from build123d import *

# Parameters (mm, degrees)
BOSS_EXTRUDE1_DEPTH = 17.018
BOSS_EXTRUDE2_DEPTH = 2.54
BOSS_EXTRUDE3_DEPTH = 6.35
SKETCH4_4_R         = 2.75
BOSS_EXTRUDE4_DEPTH = 10.414


with BuildPart() as part:
    # Sketch2 → Boss-Extrude1 (new body)
    with BuildSketch(Plane(origin=(0, 0, 0), x_dir=(1, 0, 0), z_dir=(0, 1, 0))):
        with BuildLine():
            Line((1.5, 0), (21.5, 0))
            ThreePointArc((21.5, 0), (22.560660172, -0.439339828), (23, -1.5))
            Line((23, -1.5), (23, -11.5))
            ThreePointArc((23, -11.5), (22.560660172, -12.560660172), (21.5, -13))
            Line((21.5, -13), (1.5, -13))
            ThreePointArc((1.5, -13), (0.439339828, -12.560660172), (0, -11.5))
            Line((0, -11.5), (0, -1.5))
            ThreePointArc((0, -1.5), (0.439339828, -0.439339828), (1.5, 0))
        make_face()
    extrude(amount=BOSS_EXTRUDE1_DEPTH)

    # Sketch3 → Boss-Extrude2 (add)
    with BuildSketch(Plane(origin=(0, 17.018, 0), x_dir=(1, 0, 0), z_dir=(0, 1, 0))):
        with BuildLine():
            Line((21.5, 0), (1.5, 0))
            ThreePointArc((1.5, 0), (0.439339828, -0.439339828), (0, -1.5))
            Line((0, -1.5), (0, -11.5))
            ThreePointArc((0, -11.5), (0.439339828, -12.560660172), (1.5, -13))
            Line((1.5, -13), (21.5, -13))
            ThreePointArc((21.5, -13), (22.560660172, -12.560660172), (23, -11.5))
            Line((23, -11.5), (23, -1.5))
            ThreePointArc((23, -1.5), (22.560660172, -0.439339828), (21.5, 0))
        make_face()
        with BuildLine():
            Line((0, -11.5), (0, -6.5))
            ThreePointArc((0, -6.5), (-0.557961582, -7.847038418), (-1.905, -8.405))
            Line((-1.905, -8.405), (-3.359, -8.405))
            Line((-3.359, -8.405), (-3.359, -11.5))
            ThreePointArc((-3.359, -11.5), (-2.919660172, -12.560660172), (-1.859, -13))
            Line((-1.859, -13), (1.5, -13))
            ThreePointArc((1.5, -13), (0.439339828, -12.560660172), (0, -11.5))
        make_face()
        with BuildLine():
            Line((1.5, 0), (-1.859, 0))
            ThreePointArc((-1.859, 0), (-2.919660172, -0.439339828), (-3.359, -1.5))
            Line((-3.359, -1.5), (-3.359, -4.595))
            Line((-3.359, -4.595), (-1.905, -4.595))
            ThreePointArc((-1.905, -4.595), (-0.557961582, -5.152961582), (0, -6.5))
            Line((0, -6.5), (0, -1.5))
            ThreePointArc((0, -1.5), (0.439339828, -0.439339828), (1.5, 0))
        make_face()
        with BuildLine():
            ThreePointArc((24.905, -8.405), (23.557961582, -7.847038418), (23, -6.5))
            Line((23, -6.5), (23, -11.5))
            ThreePointArc((23, -11.5), (22.560660172, -12.560660172), (21.5, -13))
            Line((21.5, -13), (24.859, -13))
            ThreePointArc((24.859, -13), (25.919660172, -12.560660172), (26.359, -11.5))
            Line((26.359, -11.5), (26.359, -8.405))
            Line((26.359, -8.405), (24.905, -8.405))
        make_face()
        with BuildLine():
            Line((24.859, 0), (21.5, 0))
            ThreePointArc((21.5, 0), (22.560660172, -0.439339828), (23, -1.5))
            Line((23, -1.5), (23, -6.5))
            ThreePointArc((23, -6.5), (23.557961582, -5.152961582), (24.905, -4.595))
            Line((24.905, -4.595), (26.359, -4.595))
            Line((26.359, -4.595), (26.359, -1.5))
            ThreePointArc((26.359, -1.5), (25.919660172, -0.439339828), (24.859, 0))
        make_face()
    extrude(amount=BOSS_EXTRUDE2_DEPTH)

    # Sketch4 → Boss-Extrude3 (add)
    with BuildSketch(Plane(origin=(0, 19.558, 0), x_dir=(1, 0, 0), z_dir=(0, 1, 0))):
        with BuildLine():
            Line((1.5, 0), (21.5, 0))
            ThreePointArc((21.5, 0), (22.560660172, -0.439339828), (23, -1.5))
            Line((23, -1.5), (23, -11.5))
            ThreePointArc((23, -11.5), (22.560660172, -12.560660172), (21.5, -13))
            Line((21.5, -13), (1.5, -13))
            ThreePointArc((1.5, -13), (0.439339828, -12.560660172), (0, -11.5))
            Line((0, -11.5), (0, -1.5))
            ThreePointArc((0, -1.5), (0.439339828, -0.439339828), (1.5, 0))
        make_face()
    extrude(amount=BOSS_EXTRUDE3_DEPTH)

    # Sketch4_4 → Boss-Extrude4 (add)
    with BuildSketch(Plane(origin=(0, 19.558, 0), x_dir=(1, 0, 0), z_dir=(0, 1, 0))):
        with Locations(Location((17.158, -6.5, 0), (0, 0, 270))):
            Circle(SKETCH4_4_R)
    extrude(amount=BOSS_EXTRUDE4_DEPTH)


solid = part.part
Input: part model. Units: mm. Frame: model coordinates. A direction names the side the tool comes from. Give positions to 0.01 mm unless a question says otherwise; leave off trailing zeros. Order: outer loops, then holes, each group sorted by start corner. A loop starts at its lowest first (then second) coordinate and runs counter-clockwise, first axis right, second up. Notation, with made-up numbers: M -1,-2 L 51,-2 A21 ccw 51,17 Z; hole C 71.25,31.25 d1. An arc over 180 degrees is marked long. Answer as a JSON object with one key per item and string values.
1. Cut plane B-B, the plane y = 16.5. Output: boundary loops of the cut face in (x, z).
Result sheet:
{"outline": "M 0,1.5 A1.5 ccw 1.5,0 L 21.5,0 A1.5 ccw 23,1.5 L 23,11.5 A1.5 ccw 21.5,13 L 1.5,13 A1.5 ccw 0,11.5 Z"}
2. Reachability of faces 4 (the flat face through (0, 23, 7)), 5 (the cylindrical face through (0.45, 8.39, 12.57)), 6 (the cylindrical face through (22.55, 22.69, 0.43)) from +Z, -Z, +X, -X, +Y, -Y: full face, straight path, thin tool, end or side. Return the list, or none.
Result sheet:
{"face 4": "+Z, -Z, -X, +Y", "face 5": "+Z, -X, -Y", "face 6": "-Z, +X, +Y"}
3. Cut plane D-D, the plane z = 7.25. Output: boundary loops of the cut face in (x, y).
Result sheet:
{"outline": "M -0.15,17.02 L 0,17.02 L 0,0 L 23,0 L 23,17.02 L 23.15,17.02 L 23.15,19.56 L 23,19.56 L 23,25.91 L 19.8,25.91 L 19.8,29.97 L 14.51,29.97 L 14.51,25.91 L 0,25.91 L 0,19.56 L -0.15,19.56 Z"}
4. First-contact query: P1, Ø1.5, axis at x = -1, z = 2, coming from the +Y side; P2, Ø3, axis at y = 24, z = 7.5, coming from the -X side; P3, Ø2, axis at y = 4, z = 8.5, coming from the +X side. Flat tips, straight axial feed; report the tip coordinate or a pass-through.
Result sheet:
{"P1": "y = 19.56", "P2": "x = 0", "P3": "x = 23"}
5. Pull-direction query (Z, two-part tool) for faces 1 (the flat face through (26.359, 18, 10)), 2 (the flat face through (26, 18, 4.595)), 3 (the cylindrical face through (22.55, 8.39, 0.43)); classes: +Z half, -Z half, draft (parallel to the pull), parting line (faces both ways), or undercut.
Result sheet:
{"face 1": "draft", "face 2": "undercut", "face 3": "-Z half"}
6. Cut plane C-C, the plane x = 12. Output: boundary loops of the cut face in (y, z), and give its area (3 significant figures).
Result sheet:
{"outline": "M 0,0 L 25.91,0 L 25.91,13 L 0,13 Z", "area": "337 mm²"}
7. Cut plane A-A, the plane z = 10. Output: boundary loops of the cut face in (x, y), and give its area (3 significant figures).
Result sheet:
{"outline": "M -3.36,17.02 L 0,17.02 L 0,0 L 23,0 L 23,17.02 L 26.36,17.02 L 26.36,19.56 L 23,19.56 L 23,25.91 L 0,25.91 L 0,19.56 L -3.36,19.56 Z", "area": "613 mm²"}
8. Ray query, line 1 (Y direction, x = 20.5, z = 1.5); line 2 (Y direction, x = 25.25, z = 3.75); line 3 (X direction, y = 22.5, z = 3.25). Return the intervals inside material, ascending. Write a range as [from, to].
Result sheet:
{"line 1": "[0, 25.91]", "line 2": "[17.02, 19.56]", "line 3": "[0, 23]"}
